Geometry: final body of the model. Coordinates: model frame, mm. A direction names the side the tool comes from. Give positions to 0.01 mm unless a question says otherwise; leave off trailing zeros. Order: outer loops, then holes, each group sorted by start corner. A loop starts at its lowest first (then second) coordinate and runs counter-clockwise, first axis right, second up. Notation, with made-up numbers: (-7.5, 69.5) -> (2.5, 69.5) arc R4 cw to (2.5, 73.5) -> close; hole circle Ø1 at (49, 11). An arc over 180 degrees is marked (long way). Write item = value, one per line.
```python
from build123d import *

# Parameters (mm, degrees)
CROQUIS1_R              = 12.5
SALIENTE_EXTRUIR1_DEPTH = 10
CORTAR_EXTRUIR1_DEPTH   = 21.310096012
MATRIZC1_COUNT          = 19
MATRIZC1_ANGLE          = 342
CORTAR_EXTRUIR2_DEPTH   = 10


with BuildPart() as part:
    # Croquis1 → Saliente-Extruir1 (new body)
    with BuildSketch(Plane.XY):
        Circle(CROQUIS1_R)
    extrude(amount=SALIENTE_EXTRUIR1_DEPTH)

    # Croquis2 → Cortar-Extruir1 (cut, through all)
    with BuildSketch(Plane(origin=(0, 0, 0), x_dir=(-1, 0, 0), z_dir=(0, 0, -1))):
        Polygon((-1.66896446, 12.5), (-0.871074147, 9.25), (0.68103554, 9.25), (1.478925853, 12.5), align=None)
    cortar_extruir1 = extrude(amount=-CORTAR_EXTRUIR1_DEPTH, mode=Mode.SUBTRACT)

    # MatrizC1: Cortar-Extruir1 ×19 about axis
    matrizc1_axis = Axis((0, 0, 0), (0, 0, 1))
    for i in range(1, MATRIZC1_COUNT):
        add(cortar_extruir1.rotate(matrizc1_axis, i * MATRIZC1_ANGLE / (MATRIZC1_COUNT - 1)), mode=Mode.SUBTRACT)

    # Croquis3 → Cortar-Extruir2 (cut)
    with BuildSketch(Plane(origin=(0, 0, 0), x_dir=(-1, 0, 0), z_dir=(0, 0, -1))):
        with BuildLine():
            Line((-1.25, 3.799671038), (-1.25, 5.25))
            Line((-1.25, 5.25), (1.25, 5.25))
            Line((1.25, 5.25), (1.25, 3.799671038))
            ThreePointArc((1.25, 3.799671038), (0, -4), (-1.25, 3.799671038))
        make_face()
    extrude(amount=-CORTAR_EXTRUIR2_DEPTH, mode=Mode.SUBTRACT)


solid = part.part
```
1) Reachability of faces 1 (the face through (2.33, 10.61, 4.93)), 2 (the face through (7.703, -9.845, 4.93)), 3 (the face through (-8.406, 6.964, 4.93)) from +Z, -Z, +X, -X, +Y, -Y: full face, straight path, thin tool, end or side. Return the list, or none.
Check sheet entries:
face_1 = +Z, -Z
face_2 = +Z, -Z, +X, -Y
face_3 = +Z, -Z, -X
2) Mould query, pull axis Y, two halves, no side actions, for faces 4 (the face through (-6.205, -8.981, 4.93)), 5 (the face through (1.26, 10.84, 4.93)), 6 (the face through (10.858, 0.307, 4.93)). Classes: +Y half, -Y half, draft (parallel to the pull), parting line (faces both ways), or undercut.
Check sheet entries:
face_4 = -Y half
face_5 = +Y half
face_6 = undercut
3) First-contact query: P1, Ø1.2, axis at x = -0.5, z = 4.5, coming from the -Y side; P2, Ø5, axis at x = -8.5, z = 6.5, coming from the +Y side; P3, Ø1.6, axis at y = 4.5, z = 5.5, coming from the +X side; P4, Ø1.6, axis at y = 4.5, z = 2.5, coming from the -X side. Flat tips, straight axial feed; report the tip coordinate or a pass-through.
Check sheet entries:
P1 = -12.5
P2 = 10.97
P3 = 11.61
P4 = -11.63
4) Line query: line 1 (Y direction, x = 0, z = 2.75); line 2 (X direction, y = 0, z = 6.5); line 3 (Y direction, x = -8, z = 4). Output: solid intervals per line, ascending. Write a range as from..to.
Check sheet entries:
line_1 = -12.5..-4, 5.25..9.25
line_2 = -9.29..-4, 4..9.27
line_3 = -9.6..-9.4, -6.03..4.66, 6.53..8.26
5) Section query A-A (x = 0). Output: boundary loops of the cut face in (y, z), plus the area to 3 significant figures.
Check sheet entries:
outline = (-12.5, 0) -> (-4, 0) -> (-4, 10) -> (-12.5, 10) -> close; (5.25, 0) -> (9.25, 0) -> (9.25, 10) -> (5.25, 10) -> close
area = 125 mm²
